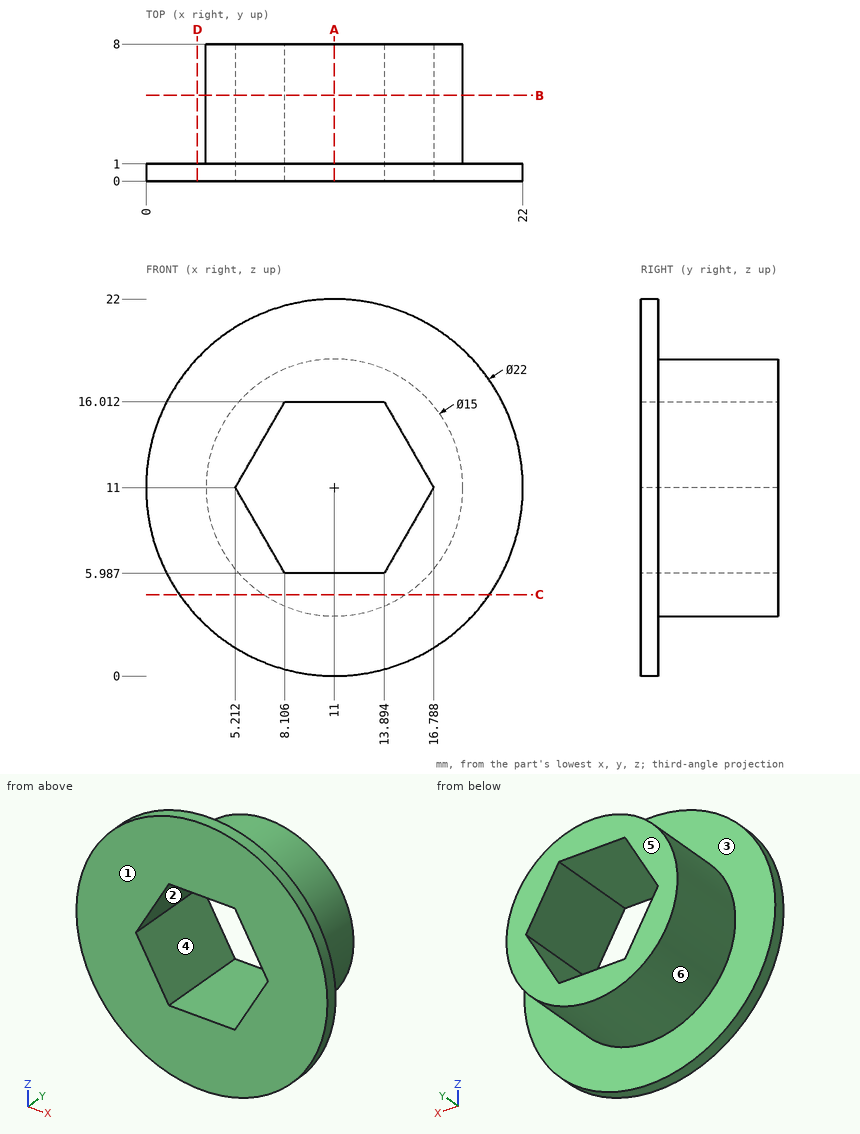
Answer from the drawing. Dimensions are ordinates in mm from the lowest x, y and z of the part. A direction names the side the tool comes from. Give positions to 0.01 mm unless a question says otherwise; leave off trailing zeros. Loops run counter-clockwise (first coordinate to the right, second up) from the corner with the lowest first, then second, coordinate; pieces in that order, holes last. Notation, with made-up numbers: (-1.75, 74.5) -> (9.25, 74.5) arc R21 ccw to (9.25, 104.5) -> close; hole circle Ø6 at (41.25, -16.75). An arc over 180 degrees is marked (long way). Use a Markdown table: item, result.
Q1. Section A-A, the plane x = 11 is taken. Determine the outline of the cut face in (y, z).
Solved:
| item | result |
|---|---|
| outline | (0, 0) -> (1, 0) -> (1, 3.5) -> (8, 3.5) -> (8, 5.99) -> (0, 5.99) -> close; (0, 16.01) -> (8, 16.01) -> (8, 18.5) -> (1, 18.5) -> (1, 22) -> (0, 22) -> close |
Q2. Determine the mould class of the marked faces 4, 5 and 6 for opening direction Z: pulls with the +Z half, pulls with the -Z half, needs draft (parallel to the pull), parting line crosses it, or undercut.
Solved:
| item | result |
|---|---|
| face 4 | undercut |
| face 5 | needs draft |
| face 6 | parting line crosses it |
Q3. Find the intervals of material crossed by line 1 along Y through (x, z) = (12.75, 20.75); line 2 along Z through (x, y) = (14.5, 1.5) (1 decimal); line 3 along Z through (x, y) = (12.75, 2.75), in increasing order.
Solved:
| item | result |
|---|---|
| line 1 | y = 0 to 1 |
| line 2 | z = 4.4 to 7, 15 to 17.6 |
| line 3 | z = 3.71 to 5.99, 16.01 to 18.29 |
Q4. Each of these flat-tipped pins is pushed along its axis until it touches: pin 1 (3 mm diameter, centred on y = 3, z = 18.5, fed in from -X); pin 2 (2 mm diameter, centred on y = 4.5, z = 15.5, fed in from -X); pin 3 (2 mm diameter, centred on y = 7, z = 8, fed in from +X). Where does it stop, or does it pass through?
Solved:
| item | result |
|---|---|
| pin 1 | stops at x = 6.5 |
| pin 2 | stops at x = 4.37 |
| pin 3 | stops at x = 18.23 |
Q5. Section D-D, the plane x = 3 is taken. Determine the outline of the cut face in (y, z), then the cut area to 3 significant figures.
Solved:
| item | result |
|---|---|
| outline | (0, 3.45) -> (1, 3.45) -> (1, 18.55) -> (0, 18.55) -> close |
| area | 15.1 mm^2 |
Q6. Section B-B, the plane y = 5 is taken. Determine the outline of the cut face in (x, z).
Solved:
| item | result |
|---|---|
| outline | circle Ø15 at (11, 11); hole (5.21, 11) -> (8.11, 5.99) -> (13.89, 5.99) -> (16.79, 11) -> (13.89, 16.01) -> (8.11, 16.01) -> close |
Q7. A tool of negligible diameter and unlimited length cuts with its end or side. For the marked faces 1, 2 and 3, from which of +Z, -Z, +X, -X, +Y, -Y can it reach the whole face along a straight path? Write none if from no direction.
Solved:
| item | result |
|---|---|
| face 1 | +Z, -Z, +X, -X, -Y |
| face 2 | +Y, -Y |
| face 3 | +Y |
Q8. Section C-C, the plane z = 4.75 is taken. Determine the outline of the cut face in (x, y) (1 decimal).
Solved:
| item | result |
|---|---|
| outline | (1.9, 0) -> (20.1, 0) -> (20.1, 1) -> (15.1, 1) -> (15.1, 8) -> (6.9, 8) -> (6.9, 1) -> (1.9, 1) -> close |
